from build123d import *

# Parameters (mm, degrees)
BOSS_EXTRUDE1_DEPTH                                 = 390
CBORE_FOR_M4_HEX_SOCKET_HEAD_CAP_SCREW3_D           = 4.5
CBORE_FOR_M4_HEX_SOCKET_HEAD_CAP_SCREW3_CBORE_D     = 8
CBORE_FOR_M4_HEX_SOCKET_HEAD_CAP_SCREW3_CBORE_DEPTH = 4.4


with BuildPart() as part:
    # esboco-convertido → Boss-Extrude1 (new body)
    with BuildSketch(Plane.XY):
        with BuildLine():
            Line((-5.17, 15), (-5.45, 14.72))
            ThreePointArc((-5.45, 14.72), (-6.002972259, 13.601894134), (-7.15, 13.111724361))
            Line((-7.15, 13.111724361), (-7.43, 12.831724361))
            Line((-7.43, 12.831724361), (-7.43, 11.562021626))
            Line((-7.43, 11.562021626), (-7.15, 11.282021626))
            ThreePointArc((-7.15, 11.282021626), (-5.99259296, 10.781953917), (-5.447208, 9.645198))
            Line((-5.447208, 9.645198), (-4.73, 8.92799))
            Line((-4.73, 8.92799), (-4.73, 6.97))
            Line((-4.73, 6.97), (-7.5, 4.2))
            Line((-7.5, 4.2), (-7.5, 0.7))
            Line((-7.5, 0.7), (-6.8, 0))
            Line((-6.8, 0), (6.8, 0))
            Line((6.8, 0), (7.5, 0.7))
            Line((7.5, 0.7), (7.5, 4.2))
            Line((7.5, 4.2), (4.73, 6.97))
            Line((4.73, 6.97), (4.73, 8.92799))
            Line((4.73, 8.92799), (5.447208, 9.645198))
            ThreePointArc((5.447208, 9.645198), (5.99259296, 10.781953917), (7.15, 11.282021626))
            Line((7.15, 11.282021626), (7.43, 11.562021626))
            Line((7.43, 11.562021626), (7.43, 12.831724361))
            Line((7.43, 12.831724361), (7.15, 13.111724361))
            ThreePointArc((7.15, 13.111724361), (6.002972259, 13.601894134), (5.45, 14.72))
            Line((5.45, 14.72), (5.17, 15))
            Line((5.17, 15), (-5.17, 15))
        make_face()
    extrude(amount=BOSS_EXTRUDE1_DEPTH)

    # CBORE for M4 Hex Socket Head Cap Screw3 (through all)
    with Locations(Plane(origin=(0, 15, 0), x_dir=(1, 0, 0), z_dir=(0, 1, 0))):
        with Locations((0, -15), (0, -375), (0, -315), (0, -255), (0, -195), (0, -135), (0, -75)):
            CounterBoreHole(CBORE_FOR_M4_HEX_SOCKET_HEAD_CAP_SCREW3_D / 2, CBORE_FOR_M4_HEX_SOCKET_HEAD_CAP_SCREW3_CBORE_D / 2, CBORE_FOR_M4_HEX_SOCKET_HEAD_CAP_SCREW3_CBORE_DEPTH)


solid = part.part
Check sheet for the modelled part. Datum: model origin and axes. Units: mm. A direction names the side the tool comes from. Coordinates: 2 decimals unless noted, no trailing zeros. Loops run counter-clockwise (first coordinate to the right, second up) from the corner with the lowest first, then second, coordinate; pieces in that order, holes last. Notation, with made-up numbers: (-21.5, 74.25) -> (-12.5, 74.25) arc R6 cw to (-12.5, 83.25) -> close; hole circle Ø2 at (19, -3.5). An arc over 180 degrees is marked (long way). Answer in a Markdown table with one row per item.
1. Access from +Z, -Z, +X, -X, +Y, -Y to the whole of each face (thin tool, end or side, straight path). Record for faces 4 (the face through (0, 0, 192)), 5 (the face through (-0.521, 12.831, 11.034)).
Check values:
| item | result |
|---|---|
| face 4 | +Z, -Z, +X, -X, -Y |
| face 5 | +Y |
2. Sectioned sample at B-B, the plane x = 0. Give the number of separate pieces and of enclosed holes in the cut face, then the cut area to 3 significant figures.
Check values:
| item | result |
|---|---|
| separate pieces | 8 |
| enclosed holes | 0 |
| area | 5,270 mm2 |
3. Material ranges on line 1 along X through (y, z) = (7.5, 195.5); line 2 along X through (y, z) = (12.4, 255); line 3 along X through (y, z) = (7, 65.5), recorded low to high. Write a range as [from, to].
Check values:
| item | result |
|---|---|
| line 1 | x = [-4.73, -2.19], [2.19, 4.73] |
| line 2 | x = [-7.43, -4], [4, 7.43] |
| line 3 | x = [-4.73, 4.73] |
4. Release check for a two-part mould opening along Z. For faces 1 (the face through (0, 8, 0)), 2 (the face through (2, 10.6, 257)), 3 (the face through (4, 15, 192)) record: released by +Z, released by -Z, zero draft, split by the parting line, or undercut.
Check values:
| item | result |
|---|---|
| face 1 | released by -Z |
| face 2 | undercut |
| face 3 | zero draft |
5. Go/stop test with flat-tipped pins: pin 1 (6 mm diameter, centred on y = 13, z = 120.5, fed in from -X); pin 2 (9 mm diameter, centred on x = 0.5, z = 133, fed in from +Y); pin 3 (4 mm diameter, centred on x = 0.5, z = 75.5, fed in from +Y); pin 4 (4 mm diameter, centred on x = 0, z = 15, fed in from -Y). Record where each tip stops, or that it passes through.
Check values:
| item | result |
|---|---|
| pin 1 | stops at x = -7.43 |
| pin 2 | stops at y = 15 |
| pin 3 | stops at y = 10.6 |
| pin 4 | passes through |
6. Sectioned sample at A-A, the plane z = 362. Record the boundary of the cut face in (x, y).
Check values:
| item | result |
|---|---|
| outline | (-7.5, 0.7) -> (-6.8, 0) -> (6.8, 0) -> (7.5, 0.7) -> (7.5, 4.2) -> (4.73, 6.97) -> (4.73, 8.93) -> (5.45, 9.65) arc R1.8 cw to (7.15, 11.28) -> (7.43, 11.56) -> (7.43, 12.83) -> (7.15, 13.11) arc R1.8 cw to (5.45, 14.72) -> (5.17, 15) -> (-5.17, 15) -> (-5.45, 14.72) arc R1.8 cw to (-7.15, 13.11) -> (-7.43, 12.83) -> (-7.43, 11.56) -> (-7.15, 11.28) arc R1.8 cw to (-5.45, 9.65) -> (-4.73, 8.93) -> (-4.73, 6.97) -> (-7.5, 4.2) -> close |
